Autodesk Inventor part; units mm, degrees
ref_plane "YZ Plane" through (0, 0, 0) normal (1, 0, 0) x (0, 1, 0)
ref_plane "XZ Plane" through (0, 0, 0) normal (0, 1, 0) x (-1, 0, 0)
ref_plane "XY Plane" through (0, 0, 0) normal (0, 0, 1) x (1, 0, 0)
sketch "Sketch1" plane through (0, 0, 0) normal (0, 0, 1) x (1, 0, 0)
  line L0 (0, 0) -> (25, 0)
  line L1 (25, 0) -> (25, 40)
  line L2 (25, 40) -> (0, 40)
  line L3 (0, 40) -> (0, 0)
  dimension "d1" = 25
  dimension "d2" = 40
  dimension "d3" = 25
extrude "Extrusion1" add sketch "Sketch1" against normal blind 30
sketch "Sketch2" plane through (25, 0, 0) normal (1, 0, 0) x (0, 0, -1)
  line L0 (0, 0) -> (30, 0)
  circle A0 centre (15, 6.56) radius 2.46
extrude "Extrusion2" cut sketch "Sketch2" against normal blind 30
sketch "Sketch3" plane through (0, 0, 0) normal (-1, 0, 0) x (0, 0, 1)
  line L0 (0, 0) -> (-30, 0)
  line L1 (-25.05, 0) -> (-4.95, 0)
  line L2 (-4.95, 0) -> (-4.95, 33.12)
  line L3 (-4.95, 33.12) -> (-25.05, 33.12)
  line L4 (-25.05, 33.12) -> (-25.05, 0)
  dimension "d11" = 20.1
extrude "Extrusion3" cut sketch "Sketch3" against normal blind 20
sketch "Sketch4" plane through (0, 0, 0) normal (0, -1, 0) x (1, 0, 0)
  line L0 (20, -4.95) -> (20, -25.05)
  line L1 (20, -15) -> (25, -15)
  line L2 (25, 0) -> (25, -30)
  line L3 (20, -8.025) -> (25, -8.025)
  line L4 (25, -8.025) -> (25, -21.975)
  line L5 (25, -21.975) -> (20, -21.975)
  line L6 (20, -21.975) -> (20, -8.025)
  line L7 (20, -8.025) -> (25, -21.975) construction
  line L8 (25, -8.025) -> (20, -21.975) construction
  line L9 (25, -12.54) -> (25, -17.46)
  point P0 (0, 0)
  point P1 (22.5, -15)
  dimension "d14" = 13.95
extrude "Extrusion4" add sketch "Sketch4" along normal blind 15
sketch "Sketch5" plane through (20, 0, 0) normal (-1, 0, 0) x (0, 0, 1)
  circle A0 centre (-15, 6.56) radius 2.46
  circle A1 centre (-15, 6.56) radius 4.7025
  circle A2 centre (-15, 6.56) radius 2.46
  circle A3 centre (-15, 6.56) radius 2.46
  point P0 (0, 0)
  dimension "d17" = 9.405
extrude "Extrusion5" cut sketch "Sketch5" against normal blind 2.1
sketch "Sketch6" plane through (25, 0, 0) normal (1, 0, 0) x (0, 0, -1)
  circle A0 centre (15, 6.56) radius 4.7025
  line L0 (15, 6.56) -> (15, 23.56)
  circle A1 centre (15, 23.56) radius 2.46
  point P0 (0, 0)
  dimension "d20" = 17
  dimension "d21" = 4.92
extrude "Extrusion6" cut sketch "Sketch6" against normal blind 10 contours A1
sketch "Sketch7" plane through (20, 0, 0) normal (-1, 0, 0) x (0, 0, 1)
  circle A0 centre (-15, 23.56) radius 2.46
  circle A1 centre (-15, 23.56) radius 4.7025
  point P0 (0, 0)
  dimension "d24" = 9.405
extrude "Extrusion7" cut sketch "Sketch7" against normal blind 2.1
sketch "Sketch9" plane through (25, 0, 0) normal (1, 0, 0) x (0, 0, -1)
  circle A0 centre (15, 6.56) radius 2.46
  circle A1 centre (15, 6.56) radius 2.46
  circle A2 centre (15, 23.56) radius 2.46
  circle A3 centre (15, 23.56) radius 2.46
  line L0 (30, 40) -> (30, 0)
  line L1 (30, 0) -> (30, 40)
  line L2 (30, 40) -> (0, 40)
  line L3 (0, 40) -> (0, 0)
  line L4 (0, 0) -> (8.025, 0)
  line L5 (21.975, 0) -> (21.975, -15)
  line L6 (21.975, -15) -> (8.025, -15)
  line L7 (8.025, -15) -> (8.025, 0)
  line L8 (0, 0) -> (8.025, 0)
  line L9 (21.975, 0) -> (30, 0)
extrude "Extrusion8" add sketch "Sketch9" along normal blind 5
sketch "Sketch10" plane through (0, 40, 0) normal (0, 1, 0) x (1, 0, 0)
  line L0 (0, 30) -> (30, 30)
  line L1 (30, 0) -> (0, 0)
  line L2 (0, 30) -> (30, 30)
  line L3 (30, 30) -> (30, 0)
  line L4 (30, 0) -> (0, 0)
  line L5 (0, 0) -> (0, 30)
extrude "Extrusion9" add sketch "Sketch10" along normal blind 30
sketch "Sketch12" plane through (30, 0, 0) normal (1, 0, 0) x (0, 0, -1)
  circle A0 centre (15, 6.56) radius 2.46
  line L0 (15, 6.56) -> (15, 15.06)
  circle A1 centre (15, 15.06) radius 2.525
  point P0 (0, 0)
  dimension "d31" = 8.5
  dimension "d33" = 5.05
extrude "Extrusion10" cut sketch "Sketch12" against normal blind 30 contours A1
sketch "Sketch14" plane through (0, 0, 0) normal (0, 0, 1) x (1, 0, 0)
  line L0 (30, 70) -> (0, 70)
  line L1 (0, 70) -> (0, 85)
  line L2 (30, 0) -> (30, 70)
  line L3 (30, 122.5) -> (30, 70)
  line L4 (30, 105) -> (30, 100)
  line L5 (-12, 153) -> (15, 153)
  line L6 (-7, 150.5) -> (-12, 153)
  line L7 (-7, 102.5) -> (-12, 100)
  line L8 (-7, 102.5) -> (-2, 126.5)
  line L9 (-2, 126.5) -> (-7, 150.5)
  line L10 (30, 126.5) -> (15, 153)
  line L11 (30, 122.5) -> (30, 126.5)
  line L12 (0, 85) -> (0, 100)
  line L13 (0, 100) -> (-12, 100)
  point P0 (0, 0)
  dimension "d90" = 12
extrude "Extrusion12" add sketch "Sketch14" against normal blind 30
sketch "Sketch15" plane through (0, 0, -25.05) normal (-1, 0, 0) x (0, 0, 1)
  line L0 (0, 33.12) -> (20.1, 33.12)
  line L1 (20.1, 33.12) -> (20.1, 0)
  line L2 (0, 33.12) -> (20.1, 33.12)
  line L3 (20.1, 33.12) -> (20.1, 31.1)
  line L4 (20.1, 31.1) -> (0, 31.1)
  line L5 (0, 31.1) -> (0, 33.12)
  point P0 (25.05, 0)
  dimension "d57" = 2.02
extrude "Extrusion13" add sketch "Sketch15" against normal blind 20
properties part number "rec_a_48mm_x_30mm"
CAD build for the part. Positions are in the model's coordinates, mm. A direction names the side the tool comes from. Coordinates: 2 decimals unless noted, no trailing zeros. Order: outer loops, then holes, each group sorted by start corner. A loop starts at its lowest first (then second) coordinate and runs counter-clockwise, first axis right, second up. Notation, with made-up numbers: M -7.5,-31 L 28.5,-31 A24 ccw 28.5,-9 Z; hole C -18,82 d10. An arc over 180 degrees is marked long. Answer as CSV lines item,"result".
1) Flat gauge pins, fed straight in: P1, Ø8, axis at x = 23, y = -7.5, coming from the -Z side (3 decimals); P2, Ø4.5, axis at y = 9, z = -13.5, coming from the -X side; P3, Ø4.5, axis at y = 23, z = -15.5, coming from the -X side. Where does each tip first touch, or does it go through?
Verdict:
P1,"z = -21.975"
P2,"x = 20"
P3,"x = 22.1"
2) Drill centre lines: L1, parallel to Z at x = 25.5, y = 23.56; L2, parallel to Z at x = 21, y = 6; L3, parallel to Y at x = 28.5, z = -15 (3 decimals). Where is each one in solid material? Low to high. Write a range as from..to.
Verdict:
L1,"-30..-17.46, -12.54..0"
L2,"-30..-19.67, -10.33..0"
L3,"-15..4.1, 9.02..12.535, 17.585..21.1, 26.02..129.15"
3) Cut at D-D (x = 25). List the corners of the cut face in (y, z) (3 decimals).
Verdict:
outline,"M -15,-21.975 L 0,-21.975 L 0,-30 L 135.333,-30 L 135.333,0 L 0,0 L 0,-8.025 L -15,-8.025 Z; hole C 6.56,-15 d4.92; hole C 15.06,-15 d5.05; hole C 23.56,-15 d4.92"
4) Cut at A-A (z = -15). Give the number of separate pieces and of enclosed holes in the cut face, then the cut area to 3 significant figures.
Verdict:
separate pieces,"4"
enclosed holes,"0"
area,"4,020 mm2"
5) Cut at B-B (y = 23.56). List the corners of the cut face in (x, z), then the cut area to 3 significant figures.
Verdict:
outline,"M 0,-30 L 30,-30 L 30,-17.46 L 22.1,-17.46 L 22.1,-19.7 L 20,-19.7 L 20,-25.05 L 0,-25.05 Z; M 0,-4.95 L 20,-4.95 L 20,-10.3 L 22.1,-10.3 L 22.1,-12.54 L 30,-12.54 L 30,0 L 0,0 Z"
area,"439 mm2"
6) Cut at C-C (x = 8). List the corners of the cut face in (y, z), then the cut area to 3 significant figures.
Verdict:
outline,"M 0,-30 L 153,-30 L 153,0 L 0,0 L 0,-4.95 L 31.1,-4.95 L 31.1,-25.05 L 0,-25.05 Z"
area,"3,960 mm2"
7) 3-axis set-ups, long thin cutter, end or side, ignore diameter. For faces 1 (the flat face through (-6, 100, -15)), 2 (the flat face through (20, 8, -20)), 3 (the flat face through (-9.46, 101.27, -14.79)), 4 (the flat face through (25, -8, -8.025)), 5 (the flat face through (18, 0, -27)): which of +Z, -Z, +X, -X, +Y, -Y reach the whole face in a straight line?
Verdict:
face 1,"+Z, -Z, -X, -Y"
face 2,"-X, -Y"
face 3,"+Z, -Z, -X"
face 4,"+Z, +X, -X, -Y"
face 5,"-Z, +X, -X, -Y"
8) Mould opens along Y. For faces 6 (the flat face through (15, 0, -3)), 7 (the cylindrical face through (25.995, 24.502, -17.272)), 8 (the flat face through (0, 62, -15)) say: released by +Y, released by -Y, zero draft, split by the parting line, or undercut.
Verdict:
face 6,"released by -Y"
face 7,"undercut"
face 8,"zero draft"
